Work out the finished part from the listing and answer in its coordinate system (mm). Face numbers are marked on the shaded views. A direction names the side the tool comes from. Coordinates: 2 decimals unless noted, no trailing zeros. Order: outer loops, then holes, each group sorted by start corner. A loop starts at its lowest first (then second) coordinate and runs counter-clockwise, first axis right, second up. Notation, with made-up numbers: M 17,65 L 44,65 A12 cw 44,82 Z; hole C -32,35 d7. An arc over 180 degrees is marked long. Write item = value, one per line. Start each with the question number.
Q1. Determine the mould class of the marked faces 1, 2, 3 and 4 for opening direction Y: released by +Y, released by -Y, zero draft, split by the parting line, or undercut.
Q2. Each of these flat-tipped pins is pushed along its axis until it touches: P1, Ø10, axis at x = 7.5, y = 6.5, coming from the +Z side; P2, Ø8, axis at x = -5.5, y = -10.5, coming from the +Z side; P3, Ø1.5, axis at x = -9, y = -8, coming from the +Z side. Where does it stop, or does it pass through?
Q3. Find section B-B on x = -14.5. Give the vertices of the cut face in (y, z).
Q4. Find section A-A on y = -1.75. Give the vertices of the cut face in (x, z), and give its area (3 significant figures).
Q5. Straight lines are drawn through the part: line 1 along Y through (x, z) = (4, 4); line 2 along X through (y, z) = (-7.25, 5.5) (3 decimals); line 3 along Y through (x, z) = (1, 7.25). For each, find the intervals that lie inside material, in ascending order.
Q6. Find section D-D on x = -22. Give the vertices of the cut face in (y, z), and give its area (3 significant figures).
Q7. A tool of negligible diameter and unlimited length cuts with its end or side. For the marked faces 5 and 6, from which of +Z, -Z, +X, -X, +Y, -Y can it reach the whole face along a straight path? Write none if from no direction.
Q8. Find section C-C on z = 4.5. Give the number of separate pieces and of enclosed holes in the cut face, and give its area (3 significant figures).
```python
from build123d import *

# Parameters (mm, degrees)
SKETCH_W        = 65
SKETCH_H        = 30
PAD_DEPTH       = 8.1
SKETCH001_W     = 58
SKETCH001_H     = 26
POCKET_DEPTH    = 1.6
POCKET001_DEPTH = 5.5
SKETCH003_W     = 20.32
SKETCH003_H     = 5.08
SKETCH003_W_2   = 16.51
SKETCH003_H_2   = 8.89
SKETCH003_W_3   = 8.89
SKETCH003_H_3   = 8.225
SKETCH003_W_4   = 35.56
POCKET002_DEPTH = 3.5
FILLET_R        = 3


with BuildPart() as part:
    # Sketch → Pad (new body)
    with BuildSketch(Plane.XY):
        Rectangle(SKETCH_W, SKETCH_H)
    extrude(amount=PAD_DEPTH)

    # Sketch001 (on DatumPlane) → Pocket (cut)
    with BuildSketch(Plane.XY.offset(8.1)):
        Rectangle(SKETCH001_W, SKETCH001_H)
    extrude(amount=-POCKET_DEPTH, mode=Mode.SUBTRACT)

    # Sketch002 (on DatumPlane) → Pocket001 (cut)
    with BuildSketch(Plane.XY.offset(8.1)):
        Polygon((-23.315, 2.84), (-24.316925, 4.219032), (-25.938075, 3.692289), (-25.938075, 1.987711), (-24.316925, 1.460968), align=None)
        Polygon((23.315, 2.84), (24.316925, 1.460968), (25.938075, 1.987711), (25.938075, 3.692289), (24.316925, 4.219032), align=None)
    extrude(amount=-POCKET001_DEPTH, mode=Mode.SUBTRACT)

    # Sketch003 (on DatumPlane) → Pocket002 (cut)
    with BuildSketch(Plane.XY.offset(6.5)):
        with Locations((-9.95, 5.38)):
            Rectangle(SKETCH003_W, SKETCH003_H)
        with Locations((11.64, 6.015)):
            Rectangle(SKETCH003_W_2, SKETCH003_H_2)
        with Locations((19.26, -7.6225)):
            Rectangle(SKETCH003_W_3, SKETCH003_H_3)
        with Locations((-6.14, -7.32)):
            Rectangle(SKETCH003_W_4, SKETCH003_H)
    extrude(amount=-POCKET002_DEPTH, mode=Mode.SUBTRACT)

    # Fillet
    fillet_edges = [part.edges().sort_by_distance(p)[0] for p in [
        (-32.5, -15, 4.05),
        (32.5, -15, 4.05),
        (32.5, 15, 4.05),
        (-32.5, 15, 4.05),
    ]]
    fillet(fillet_edges, radius=FILLET_R)


solid = part.part
```
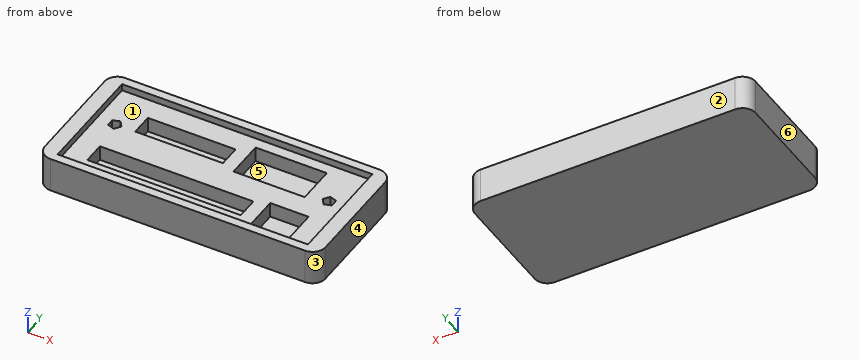
Findings below:
q1.face_1 = undercut
q1.face_2 = released by +Y
q1.face_3 = released by -Y
q1.face_4 = zero draft
q2.P1 = 6.5
q2.P2 = 8.1
q2.P3 = 3
q3.outline = M -15,0 L 15,0 L 15,8.1 L 13,8.1 L 13,6.5 L 7.92,6.5 L 7.92,3 L 2.84,3 L 2.84,6.5 L -4.78,6.5 L -4.78,3 L -9.86,3 L -9.86,6.5 L -13,6.5 L -13,8.1 L -15,8.1 Z
q4.outline = M -32.5,0 L 32.5,0 L 32.5,8.1 L 29,8.1 L 29,6.5 L -29,6.5 L -29,8.1 L -32.5,8.1 Z
q4.area = 434 mm^2
q5.line_1 = -15 to -9.86, -4.78 to 1.57, 10.46 to 15
q5.line_2 = -32.5 to -23.92, 11.64 to 14.815, 23.705 to 32.5
q5.line_3 = -15 to -13, 13 to 15
q6.outline = M -15,0 L 15,0 L 15,8.1 L 13,8.1 L 13,6.5 L -4.78,6.5 L -4.78,3 L -9.86,3 L -9.86,6.5 L -13,6.5 L -13,8.1 L -15,8.1 Z
q6.area = 184 mm^2
q7.face_5 = +Z
q7.face_6 = +Z, -Z, -X, +Y, -Y
q8.separate_pieces = 1
q8.enclosed_holes = 6
q8.area = 1,430 mm^2
